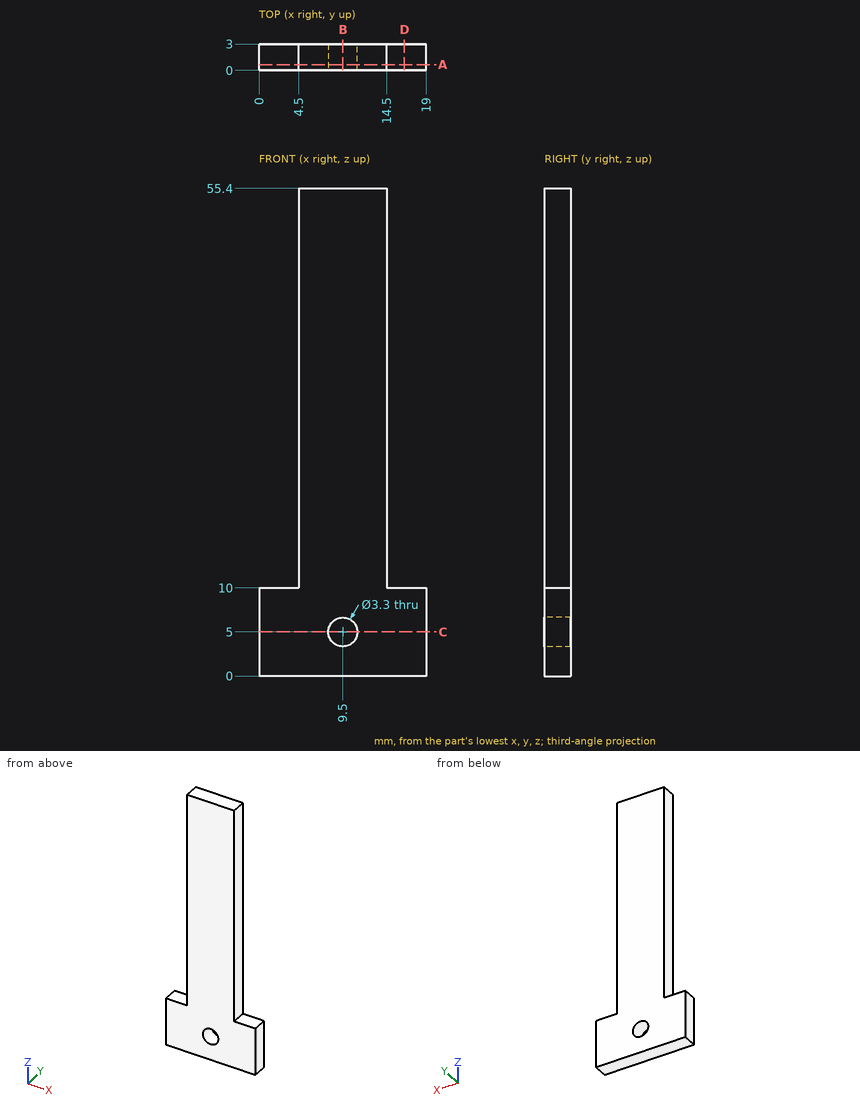
Drawing for the job (mm, zero at the part's lowest x, y, z). Give positions to 0.01 mm unless a question says otherwise; leave off trailing zeros. Loops run counter-clockwise (first coordinate to the right, second up) from the corner with the lowest first, then second, coordinate; pieces in that order, holes last.
(1) Band-saw the part on B-B (x = 9.5). Write the cut outline in (y, z), and give its area (3 significant figures).
Return value:
outline: (0, 0) - (3, 0) - (3, 3.35) - (0, 3.35) - close; (0, 6.65) - (3, 6.65) - (3, 55.4) - (0, 55.4) - close
area: 156 mm2
(2) Drill centre lines: line 1 along X through (y, z) = (1.7, 5); line 2 along Z through (x, y) = (9.5, 1.75); line 3 along X through (y, z) = (2.4, 33.5). Where is each one in solid material? Low to high.
Return value:
line 1: x = 0 to 7.85, 11.15 to 19
line 2: z = 0 to 3.35, 6.65 to 55.4
line 3: x = 4.5 to 14.5
(3) Pin check, flat tips, straight feed: pin 1 (1.5 mm diameter, centred on y = 1.5, z = 25.5, fed in from +X); pin 2 (1.5 mm diameter, centred on x = 17, y = 1.5, fed in from +Z). Stop position of each tip, or through.
Return value:
pin 1: stops at x = 14.5
pin 2: stops at z = 10
(4) Band-saw the part on D-D (x = 16.5). Write the cut outline in (y, z), and give its area (3 significant figures).
Return value:
outline: (0, 0) - (3, 0) - (3, 10) - (0, 10) - close
area: 30.0 mm2
(5) Band-saw the part on A-A (y = 0.65). Write the cut outline in (x, z), and give its area (3 significant figures).
Return value:
outline: (0, 0) - (19, 0) - (19, 10) - (14.5, 10) - (14.5, 55.4) - (4.5, 55.4) - (4.5, 10) - (0, 10) - close; hole circle Ø3.3 at (9.5, 5)
area: 635 mm2
(6) Band-saw the part on C-C (z = 5). Write the cut outline in (x, y), and give its area (3 significant figures).
Return value:
outline: (0, 0) - (7.85, 0) - (7.85, 3) - (0, 3) - close; (11.15, 0) - (19, 0) - (19, 3) - (11.15, 3) - close
area: 47.1 mm2
